Design review of the part built by this model. Coordinates are the model's own, in mm. A direction names the side the tool comes from. Give positions to 0.01 mm unless a question says otherwise; leave off trailing zeros. Loops run counter-clockwise (first coordinate to the right, second up) from the corner with the lowest first, then second, coordinate; pieces in that order, holes last. Notation, with made-up numbers: (66, -26.75) - (113, -26.75) arc R13 ccw to (113, -15.75) - close; hole circle Ø10 at (-7, -26). An arc over 180 degrees is marked (long way). Put each result on its own line as item: value. Start each with the question number.
```python
from build123d import *

# Parameters (mm, degrees)
CROQUIS1_R              = 3.5
SALIENTE_EXTRUIR1_DEPTH = 4
CROQUIS2_R              = 1.5
SALIENTE_EXTRUIR2_DEPTH = 12
CHAFL_N1_SIZE           = 0.2
CORTAR_EXTRUIR1_DEPTH   = 2


with BuildPart() as part:
    # Croquis1 → Saliente-Extruir1 (new body)
    with BuildSketch(Plane(origin=(0, 0, 0), x_dir=(1, 0, 0), z_dir=(0, 1, 0))):
        with Locations(Location((0, 0, 0), (0, 0, 270))):
            Circle(CROQUIS1_R)
    extrude(amount=SALIENTE_EXTRUIR1_DEPTH)

    # Croquis2 → Saliente-Extruir2 (add)
    with BuildSketch(Plane.XZ):
        with Locations(Location((0, 0, 0), (0, 0, 270))):
            Circle(CROQUIS2_R)
    extrude(amount=SALIENTE_EXTRUIR2_DEPTH)

    # Chaflán1
    chafl_n1_edges = [part.edges().sort_by_distance(p)[0] for p in [
        (0, -12, 1.5),
    ]]
    chamfer(chafl_n1_edges, length=CHAFL_N1_SIZE)

    # Croquis3 → Cortar-Extruir1 (cut)
    with BuildSketch(Plane(origin=(0, 4, 0), x_dir=(1, 0, 0), z_dir=(0, 1, 0))):
        Polygon((0, 2.289686923), (-1.982927042, 1.144843462), (-1.982927042, -1.144843462), (0, -2.289686923), (1.982927042, -1.144843462), (1.982927042, 1.144843462), align=None)
    extrude(amount=-CORTAR_EXTRUIR1_DEPTH, mode=Mode.SUBTRACT)


solid = part.part
```
Item 1: For L1, parallel to Y at x = -0.75, z = 1.5; L2, parallel to Y at x = -2.25, z = -0.75; L3, parallel to Z at x = -0.75, y = -0.5, list the stretches that pass through material, from the lowest coordinate up. Write a range as from..to.
Item 2: Machinability: for faces 4 (the flat face through (-1.005, 3.014, 1.709)), 5 (the flat face through (-2, 4, 2)), 6 (the flat face through (0, 0, 2)), which of the approach directions +Z, -Z, +X, -X, +Y, -Y give a long, thin tool a straight path to every point of the face, cutting with its end or side? Answer none if there is none.
Item 3: Consider section A-A (z = 0). State the section outline as (x, y) points, plus the area to 3 significant figures.
Item 4: Mouldability with a two-part tool opening along Z and no side actions: class faces 1 (the flat face through (0, -12, 0)), 2 (the flat face through (0.978, 3.014, 1.725)), 3 (the cylindrical face through (0.45, -5.82, -1.43)) as pulls with the +Z half, pulls with the -Z half, needs draft (parallel to the pull), parting line crosses it, or undercut.
Item 5: For P1, Ø1, axis at y = -2, z = 0, coming from the +X side; P2, Ø2, axis at x = 1, y = -3.5, coming from the -Z side; P3, Ø2, axis at y = -6.5, z = -2, coming from the +X side, all flat-tipped, find the tip position at first contact; note any pin that passes through.
Item 6: Consider section C-C (x = -2.5). State the section outline as (y, z) points.
Item 7: Consider section B-B (y = -10.5). State the section outline as (x, z) points, plus the area to 3 significant figures.
Item 8: Consider section D-D (z = 3). State the section outline as (x, y) points, plus the area to 3 significant figures.
Geometry says:
1. L1: y = 0..2
1. L2: y = 0..4
1. L3: z = -1.3..1.3
2. face 4: +Y
2. face 5: +Z, -Z, +X, -X, +Y
2. face 6: -Y
3. outline: (-3.5, 0) - (-1.5, 0) - (-1.5, -11.8) - (-1.3, -12) - (1.3, -12) - (1.5, -11.8) - (1.5, 0) - (3.5, 0) - (3.5, 4) - (1.98, 4) - (1.98, 2) - (-1.98, 2) - (-1.98, 4) - (-3.5, 4) - close
3. area: 56.0 mm2
4. face 1: needs draft
4. face 2: undercut
4. face 3: parting line crosses it
5. P1: stops at x = 1.5
5. P2: stops at z = -1.5
5. P3: stops at x = 1.12
6. outline: (0, -2.45) - (4, -2.45) - (4, 2.45) - (0, 2.45) - close
7. outline: circle Ø3 at (0, 0)
7. area: 7.07 mm2
8. outline: (-1.8, 0) - (1.8, 0) - (1.8, 4) - (-1.8, 4) - close
8. area: 14.4 mm2
